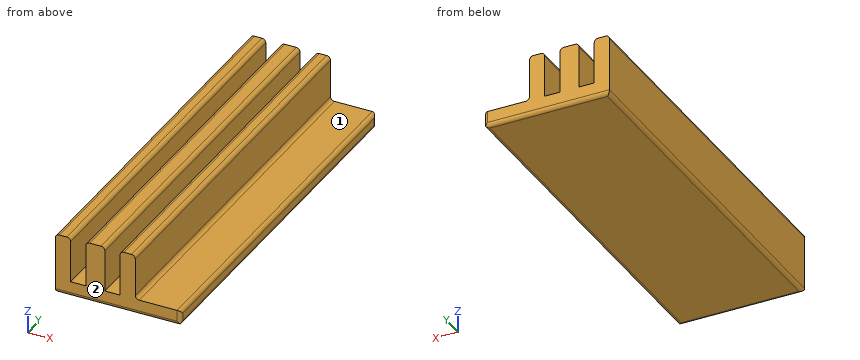
```python
from build123d import *

# Parameters (mm, degrees)
F1_DEPTH    = 50
F2_T1_DEPTH = 52.54
F2_T3_DEPTH = 4.54
F3_R        = 0.508
F4_T1_DEPTH = 18.532
F4_T3_DEPTH = 52.54
F5_R        = 0.508


# Not quite as in the source:
# - a fillet or chamfer that OpenCascade refuses, or shapes differently, is made with other operations: its cross-section is extruded or revolved along the edge and cut away or added


with BuildPart() as f1:
    # F0 (on Front) → F1 (new body)
    with BuildSketch(Plane.XZ):
        Polygon((0, 8), (0, 0), (16.5, 0), (16.5, 2), (10.5, 2), (10.5, 8), (8.5, 8), (8.5, 2), (6.5, 2), (6.5, 8), (4, 8), (4, 2), (2, 2), (2, 8), align=None)
    extrude(amount=F1_DEPTH)

    # F2: fillet of radius 0.508 on 4 edges, made by hand

    # F2_s2 → F2_t1 (cut)
    with BuildSketch(Plane.XZ.offset(-1.27)):
        with BuildLine():
            ThreePointArc((15.992, 0), (16.3512102448, 0.1487897552), (16.5, 0.508))
            Line((16.5, 0.508), (16.5, 0))
            Line((16.5, 0), (15.992, 0))
        make_face()
        with BuildLine():
            ThreePointArc((16.5, 1.492), (16.3512102448, 1.8512102448), (15.992, 2))
            Line((15.992, 2), (16.5, 2))
            Line((16.5, 2), (16.5, 1.492))
        make_face()
    extrude(amount=F2_T1_DEPTH, mode=Mode.SUBTRACT)

    # F2_s4 → F2_t3 (cut)
    with BuildSketch(Plane.XY.offset(-1.27)):
        with BuildLine():
            ThreePointArc((16.5, -0.508), (16.3512102448, -0.1487897552), (15.992, 0))
            Line((15.992, 0), (16.5, 0))
            Line((16.5, 0), (16.5, -0.508))
        make_face()
        with BuildLine():
            ThreePointArc((16.5, -49.492), (16.3512102448, -49.8512102448), (15.992, -50))
            Line((15.992, -50), (16.5, -50))
            Line((16.5, -50), (16.5, -49.492))
        make_face()
    extrude(amount=F2_T3_DEPTH, mode=Mode.SUBTRACT)

    # F3
    f3_edges = [f1.edges().sort_by_distance(p)[0] for p in [
        (8.5, -25, 8),
        (10.5, -25, 8),
        (6.5, -25, 8),
        (4, -25, 8),
        (2, -25, 8),
        (0, -25, 8),
    ]]
    fillet(f3_edges, radius=F3_R)

    # F4: fillet of radius 0.508 on 4 edges, made by hand

    # F4_s2 → F4_t1 (cut)
    with BuildSketch(Plane.YZ.offset(-1.27)):
        with BuildLine():
            ThreePointArc((0, 0.508), (-0.1487897552, 0.1487897552), (-0.508, 0))
            Line((-0.508, 0), (0, 0))
            Line((0, 0), (0, 0.508))
        make_face()
        with BuildLine():
            ThreePointArc((-49.492, 0), (-49.8512102448, 0.1487897552), (-50, 0.508))
            Line((-50, 0.508), (-50, 0))
            Line((-50, 0), (-49.492, 0))
        make_face()
    extrude(amount=F4_T1_DEPTH, mode=Mode.SUBTRACT)

    # F4_s4 → F4_t3 (cut)
    with BuildSketch(Plane.XZ.offset(-1.27)):
        with BuildLine():
            ThreePointArc((0, 0.508), (0.1487897552, 0.1487897552), (0.508, 0))
            Line((0.508, 0), (0, 0))
            Line((0, 0), (0, 0.508))
        make_face()
    extrude(amount=F4_T3_DEPTH, mode=Mode.SUBTRACT)

    # F5
    f5_edges = [f1.edges().sort_by_distance(p)[0] for p in [
        (10.5, -25, 2),
    ]]
    fillet(f5_edges, radius=F5_R)


solid = f1.part
```
Can you work these out from the model? Positions are in its coordinate system, mm. Face numbers are marked on the shaded views. A direction names the side the tool comes from. Give positions to 0.01 mm unless a question says otherwise; leave off trailing zeros. Loops run counter-clockwise (first coordinate to the right, second up) from the corner with the lowest first, then second, coordinate; pieces in that order, holes last. Notation, with made-up numbers: M 24,80 L 81,80 A15 ccw 81,101 Z; hole C 9.25,-15 d5. An arc over 180 degrees is marked long. One line per item, written item: value.
(1) Suppose I cut it at B-B on x = 13. List the corners of the cut face in (y, z) for me.
Returned:
outline: M -50,0.51 A0.51 ccw -49.49,0 L -0.51,0 A0.51 ccw 0,0.51 L 0,2 L -50,2 Z
(2) Will these pins go through, and if not, where does the flat tip stop? pin 1 (2 mm diameter, centred on x = 12.5, y = -39.5, fed in from +Z); pin 2 (5.5 mm diameter, centred on x = 13.5, y = -18, fed in from +Z); pin 3 (2.5 mm diameter, centred on y = -36.5, z = 4.5, fed in from +X); pin 4 (1.5 mm diameter, centred on y = -37, z = 2, fed in from +X).
Returned:
pin 1: z = 2
pin 2: z = 2.07
pin 3: x = 10.5
pin 4: x = 16.5
(3) I need wall thicknesses on line 1 (X direction, y = -17, z = 3); line 2 (X direction, y = -26, z = 2.25); line 3 (Z direction, x = 15.5, y = -6.5). Which ranges of each line are inside material? Lowest first, please.
Returned:
line 1: 0 to 2, 4 to 6.5, 8.5 to 10.5
line 2: 0 to 2, 4 to 6.5, 8.5 to 10.57
line 3: 0 to 2
(4) Which directions (+Z, -Z, +X, -X, +Y, -Y) give clear straight access to the entire face, cutting with the end or side of a thin tool? Please do the marked faces 1 and 2.
Returned:
face 1: +Z, +X, +Y, -Y
face 2: +Z, -Z, +X, -X, -Y
(5) Suppose I cut it at A-A on z = 3. List the corners of the cut face in (x, y) for me, plus the area to 3 significant figures.
Returned:
outline: M 0,-50 L 2,-50 L 2,0 L 0,0 Z; M 4,-50 L 6.5,-50 L 6.5,0 L 4,0 Z; M 8.5,-50 L 10.5,-50 L 10.5,0 L 8.5,0 Z
area: 325 mm^2
(6) Suppose I cut it at C-C on y = -23. List the corners of the cut face in (x, z) for me.
Returned:
outline: M 0,0.51 A0.51 ccw 0.51,0 L 15.99,0 A0.51 ccw 16.5,0.51 L 16.5,1.49 A0.51 ccw 15.99,2 L 11.01,2 A0.51 cw 10.5,2.51 L 10.5,7.49 A0.51 ccw 9.99,8 L 9.01,8 A0.51 ccw 8.5,7.49 L 8.5,2 L 6.5,2 L 6.5,7.49 A0.51 ccw 5.99,8 L 4.51,8 A0.51 ccw 4,7.49 L 4,2 L 2,2 L 2,7.49 A0.51 ccw 1.49,8 L 0.51,8 A0.51 ccw 0,7.49 Z
